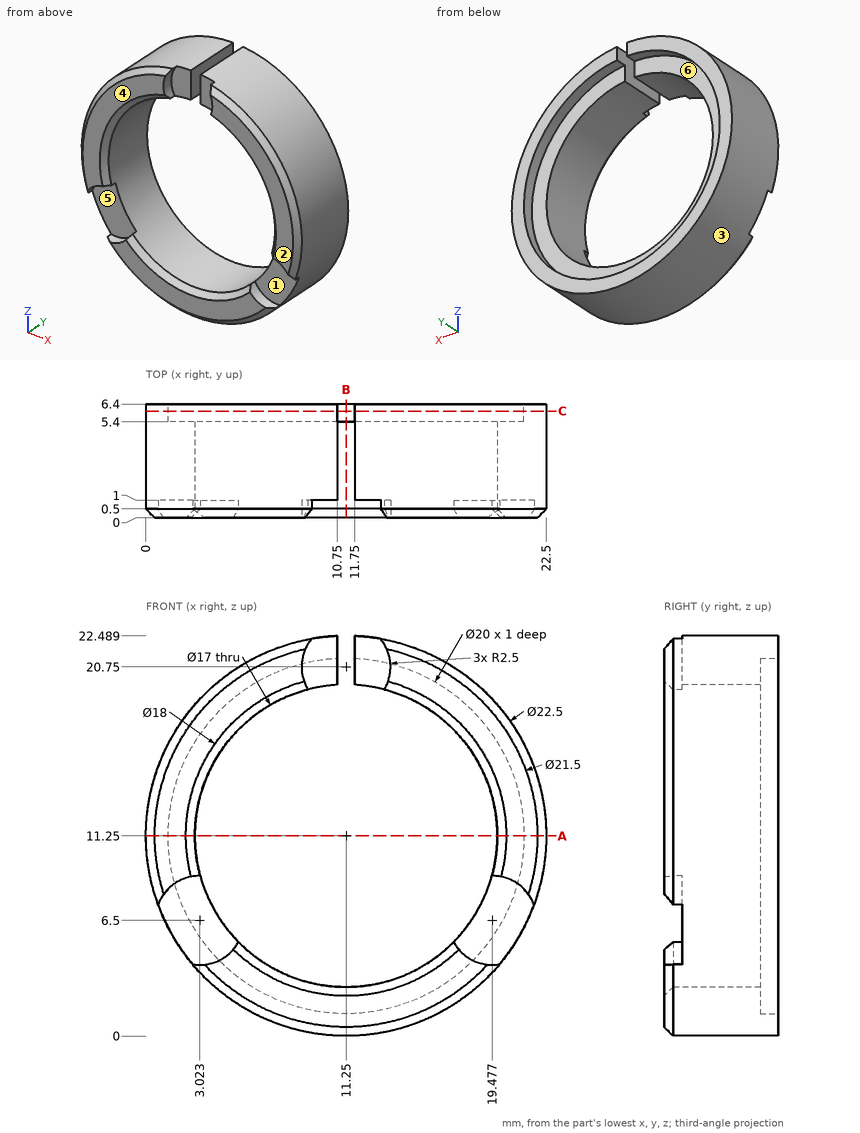
Verification items for this drawing (mm, ordinates from the low corner). A direction names the side the tool comes from. Give positions to 0.01 mm unless a question says otherwise; leave off trailing zeros. Loops run counter-clockwise (first coordinate to the right, second up) from the corner with the lowest first, then second, coordinate; pieces in that order, holes last. Notation, with made-up numbers: M 20,86.5 L 54,86.5 A15 ccw 54,115.5 Z; hole C 68.25,-6.5 d8. An arc over 180 degrees is marked long. Answer as a JSON object with one key per item and string values. Group by question number.
Item 1: Access from +Z, -Z, +X, -X, +Y, -Y to the whole of each face (thin tool, end or side, straight path). Record for the marked faces 4, 5 and 6.
Item 2: Sectioned sample at B-B on x = 11.25. Record the boundary of the cut face in (y, z).
Item 3: Mould release check, pull along Z, two halves, no side actions. Record for the marked faces 1, 2 and 3: pulls with the +Z half, pulls with the -Z half, needs draft (parallel to the pull), parting line crosses it, or undercut.
Item 4: Sectioned sample at C-C on y = 6. Record the boundary of the cut face in (x, z).
Item 5: Material ranges on L1, parallel to X at y = 1.6, z = 11.25; L2, parallel to X at y = 6.25, z = 11.25; L3, parallel to Z at x = 11.25, y = 2.5, recorded low to high.
Item 6: Sectioned sample at A-A on z = 11.25. Record the boundary of the cut face in (x, y).
Item 7: Gauge pin test, flat ends, axial feed: pin 1 (0.6 mm diameter, centred on x = 13, z = 20.5, fed in from -Y); pin 2 (1 mm diameter, centred on x = 16, y = 1, fed in from +Z); pin 3 (2 mm diameter, centred on y = 3.5, z = 20.5, fed in from -X). Record the tip position at first contact, or that the pin passes through.
Findings below:
{
 "1": {"face 4": "+Z, -Z, +X, -X, -Y", "face 5": "-Y", "face 6": "+Y"},
 "2": {"outline": "M 0,0.5 L 0.5,0 L 6.4,0 L 6.4,1.25 L 5.4,1.25 L 5.4,2.75 L 0.5,2.75 L 0,2.25 Z"},
 "3": {"face 1": "undercut", "face 2": "needs draft", "face 3": "parting line crosses it"},
 "4": {"outline": "M 10.75,21.24 L 10.75,22.49 A11.25 ccw long 11.75,22.49 L 11.75,21.24 A10 cw long Z"},
 "5": {"L1": "0 to 2.75, 19.75 to 22.5", "L2": "0 to 1.25, 21.25 to 22.5", "L3": "0 to 2.75"},
 "6": {"outline": "M 0,0.5 L 0.5,0 L 2.25,0 L 2.75,0.5 L 2.75,5.4 L 1.25,5.4 L 1.25,6.4 L 0,6.4 Z; M 19.75,0.5 L 20.25,0 L 22,0 L 22.5,0.5 L 22.5,6.4 L 21.25,6.4 L 21.25,5.4 L 19.75,5.4 Z"},
 "7": {"pin 1": "y = 1", "pin 2": "z = 21.67", "pin 3": "x = 3.6"}
}
